Here's how the part is built. I have some questions about the finished solid (model axes, mm). Give positions to 0.01 mm unless a question says otherwise; leave off trailing zeros. Write each loop counter-clockwise with the first axis right and the second up, starting at its lowest first coordinate (ties: lowest second). Pieces come first, ordered by that corner, then holes. Notation, with made-up numbers: (-6, -5.75) - (48, -5.75) arc R16 ccw to (48, -0.75) - close; hole circle Ø6 at (-38.5, 9). An arc over 180 degrees is marked (long way). Write each question's results on one line, items separated by ' | '. Start each with the question number.
Item 1: Please list where these lines run through material, in increasing order: line 1 along X through (y, z) = (0.5, 1); line 2 along X through (y, z) = (1.35, 0); line 3 along X through (y, z) = (1.35, 0.5).
Item 2: Will these pins go through, and if not, where does the flat tip stop? P1, Ø1.8, axis at x = 0.55, z = 4.7, coming from the +Y side; P2, Ø4, axis at x = -5, z = 3, coming from the -Y side; P3, Ø1, axis at x = 4, y = 1, coming from the -Z side.
Item 3: Suppose I cut it at D-D on x = -2. List the corners of the cut face in (y, z) for me.
Item 4: Suppose I cut it at A-A on z = 0. List the corners of the cut face in (x, y) for me, then the cut area to 3 significant figures.
Item 5: We'd pull the mould along X, two halves only. Please class faces 1 (the cylindrical face through (-6.834, 0.986, -1.517)), 2 (the flat face through (0, 0, 3)), 3 (the cylindrical face through (-2.44, 1.01, -0.54)): +X half, -X half, draft (parallel to the pull), parting line (faces both ways), or undercut.
Item 6: Suppose I cut it at C-C on z = 1.5. List the corners of the cut face in (x, y) for me.
Item 7: Suppose I cut it at B-B on x = 0. List the corners of the cut face in (y, z) for me, then the cut area to 3 significant figures.
```python
from build123d import *

# Parameters (mm, degrees)
SKETCH_1_R                         = 7
EXTRUDE_1_DEPTH                    = 2
SKETCH_2_R                         = 1.1
CUT_EXTRUDE_1_DEPTH                = 2
PATTERN_CIRCULAR_1_COUNT           = 2
PATTERN_CIRCULAR_1_ANGLE           = 90
PATTERN_CIRCULAR_1_COPY_1_SKETCH_R = 1.1
PATTERN_CIRCULAR_1_COPY_1_DEPTH    = 2
SKETCH_3_R                         = 2.5
CUT_EXTRUDE_2_DEPTH                = 2


with BuildPart() as part:
    # Sketch 1 → Extrude 1 (new body)
    with BuildSketch(Plane(origin=(0, 0, 0), x_dir=(1, 0, 0), z_dir=(0, 1, 0))):
        with Locations(Location((0, 0, 0), (0, 0, 270))):
            Circle(SKETCH_1_R)
    extrude(amount=EXTRUDE_1_DEPTH)

    # Sketch 2 → Cut-Extrude 1 (cut)
    with BuildSketch(Plane(origin=(0, 2, 0), x_dir=(1, 0, 0), z_dir=(0, 1, 0))):
        with Locations(Location((-0.524681621, 4.469307463, 0), (0, 0, 270))):
            Circle(SKETCH_2_R)
    cut_extrude_1 = extrude(amount=-CUT_EXTRUDE_1_DEPTH, mode=Mode.SUBTRACT)

    # Mirror 1: Cut-Extrude 1 across plane
    add(cut_extrude_1.mirror(Plane(origin=(0.013284469, 0, 0.113158862), x_dir=(0.9931794361720326, 0, -0.11659591573036844), z_dir=(0.11659591573036844, 0, 0.9931794361720327))), mode=Mode.SUBTRACT)

    # Pattern Circular 1: Cut-Extrude 1 ×2 about axis
    pattern_circular_1_axis = Axis((0.013284469, 0, 0.113158862), (0, -1, 0))
    for i in range(1, PATTERN_CIRCULAR_1_COUNT):
        add(cut_extrude_1.rotate(pattern_circular_1_axis, i * PATTERN_CIRCULAR_1_ANGLE / (PATTERN_CIRCULAR_1_COUNT - 1)), mode=Mode.SUBTRACT)

    # Pattern Circular 1 copy 1 sketch → Pattern Circular 1 copy 1 (cut)
    with BuildSketch(Plane(origin=(-0.099874394, 2, 0.126443331), x_dir=(0.23160133169009495, 0, 0.9728107848699944), z_dir=(0, 1, 0))):
        with Locations((-0.524681621, -4.469307463)):
            Circle(PATTERN_CIRCULAR_1_COPY_1_SKETCH_R)
    extrude(amount=-PATTERN_CIRCULAR_1_COPY_1_DEPTH, mode=Mode.SUBTRACT)

    # Sketch 3 → Cut-Extrude 2 (cut)
    with BuildSketch(Plane(origin=(0, 2, 0), x_dir=(1, 0, 0), z_dir=(0, 1, 0))):
        with Locations(Location((0, 0, 0), (0, 0, 270))):
            Circle(SKETCH_3_R)
    extrude(amount=-CUT_EXTRUDE_2_DEPTH, mode=Mode.SUBTRACT)


solid = part.part
```
Checked values:
1) line 1: x = -6.93 to -5.61, -3.53 to -2.29, 2.29 to 6.93 | line 2: x = -7 to -5.46, -3.68 to -2.5, 2.5 to 3.58, 5.61 to 7 | line 3: x = -6.98 to -5.66, -3.48 to -2.45, 2.45 to 4, 5.19 to 6.98
2) P1: passes through | P2: stops at y = 0 | P3: stops at z = -6.06
3) outline: (0, -6.71) - (2, -6.71) - (2, -1.5) - (0, -1.5) - close; (0, 1.5) - (2, 1.5) - (2, 6.71) - (0, 6.71) - close
4) outline: (-7, 0) - (-5.46, 0) - (-5.46, 2) - (-7, 2) - close; (-3.68, 0) - (-2.5, 0) - (-2.5, 2) - (-3.68, 2) - close; (2.5, 0) - (3.58, 0) - (3.58, 2) - (2.5, 2) - close; (5.61, 0) - (7, 0) - (7, 2) - (5.61, 2) - close | area: 10.4 mm^2
5) face 1: parting line | face 2: draft | face 3: undercut
6) outline: (-6.84, 0) - (-5.27, 0) - (-5.27, 2) - (-6.84, 2) - close; (-3.87, 0) - (-2, 0) - (-2, 2) - (-3.87, 2) - close; (2, 0) - (6.84, 0) - (6.84, 2) - (2, 2) - close
7) outline: (0, -7) - (2, -7) - (2, -5.44) - (0, -5.44) - close; (0, -3.5) - (2, -3.5) - (2, -2.5) - (0, -2.5) - close; (0, 2.5) - (2, 2.5) - (2, 3.74) - (0, 3.74) - close; (0, 5.65) - (2, 5.65) - (2, 7) - (0, 7) - close | area: 10.3 mm^2
